from build123d import *

# Parameters (mm, degrees)
SKETCH1_W           = 70
SKETCH1_H           = 41
BOSS_EXTRUDE1_DEPTH = 12
SKETCH2_W           = 50
SKETCH2_H           = 1
CUT_EXTRUDE1_DEPTH  = 88
SKETCH3_R           = 2.5
SKETCH3_R_2         = 2.75
CUT_EXTRUDE2_DEPTH  = 88
SKETCH4_R           = 5
CUT_EXTRUDE3_DEPTH  = 5.7
SKETCH5_R           = 2.5
CUT_EXTRUDE4_DEPTH  = 12
SKETCH6_R           = 6
SKETCH6_R_2         = 5.5
CUT_EXTRUDE5_DEPTH  = 39
SKETCH8_R           = 2.5
BOSS_EXTRUDE2_DEPTH = 41
SKETCH9_R           = 2.5
CUT_EXTRUDE6_DEPTH  = 12
SKETCH10_R          = 6
CUT_EXTRUDE7_DEPTH  = 30


with BuildPart() as part:
    # Sketch1 → Boss-Extrude1 (new body)
    with BuildSketch(Plane(origin=(0, 0, 0), x_dir=(1, 0, 0), z_dir=(0, 1, 0))):
        Rectangle(SKETCH1_W, SKETCH1_H)
    extrude(amount=BOSS_EXTRUDE1_DEPTH)

    # Sketch2 → Cut-Extrude1 (cut)
    with BuildSketch(Plane.XY.offset(20.5)):
        with Locations((0, 11.5)):
            Rectangle(SKETCH2_W, SKETCH2_H)
    extrude(amount=-CUT_EXTRUDE1_DEPTH, mode=Mode.SUBTRACT)

    # Sketch3 → Cut-Extrude2 (cut)
    with BuildSketch(Plane.XZ):
        with Locations((29, -7.5)):
            Circle(SKETCH3_R)
        with Locations((-29, 7.5)):
            Circle(SKETCH3_R)
        with Locations((29, 7.5)):
            Circle(SKETCH3_R_2)
        with Locations((-29, -7.5)):
            Circle(SKETCH3_R_2)
    extrude(amount=-CUT_EXTRUDE2_DEPTH, mode=Mode.SUBTRACT)

    # Sketch4 → Cut-Extrude3 (cut)
    with BuildSketch(Plane.XZ):
        with Locations((-29, -7.5)):
            Circle(SKETCH4_R)
        with Locations((29, 7.5)):
            Circle(SKETCH4_R)
    extrude(amount=-CUT_EXTRUDE3_DEPTH, mode=Mode.SUBTRACT)

    # Sketch5 → Cut-Extrude4 (cut)
    with BuildSketch(Plane(origin=(0, 0, -20.5), x_dir=(-1, 0, 0), z_dir=(0, 0, -1))):
        with Locations((-6.5, 6)):
            Circle(SKETCH5_R)
    extrude(amount=-CUT_EXTRUDE4_DEPTH, mode=Mode.SUBTRACT)

    # Sketch6 → Cut-Extrude5 (cut)
    with BuildSketch(Plane.XZ):
        Circle(SKETCH6_R)
        with Locations((-17.5, 0)):
            Circle(SKETCH6_R_2)
        with Locations((17.5, 0)):
            Circle(SKETCH6_R_2)
    extrude(amount=-CUT_EXTRUDE5_DEPTH, mode=Mode.SUBTRACT)

    # Sketch8 → Boss-Extrude2 (add)
    with BuildSketch(Plane(origin=(0, 0, -20.5), x_dir=(-1, 0, 0), z_dir=(0, 0, -1))):
        with Locations((-6.5, 6)):
            Circle(SKETCH8_R)
    extrude(amount=-BOSS_EXTRUDE2_DEPTH)

    # Sketch9 → Cut-Extrude6 (cut)
    with BuildSketch(Plane(origin=(0, 0, -20.5), x_dir=(-1, 0, 0), z_dir=(0, 0, -1))):
        with Locations((-6.5, 5.5)):
            Circle(SKETCH9_R)
    extrude(amount=-CUT_EXTRUDE6_DEPTH, mode=Mode.SUBTRACT)

    # Sketch10 → Cut-Extrude7 (cut)
    with BuildSketch(Plane(origin=(0, 11, 0), x_dir=(1, 0, 0), z_dir=(0, 1, 0))):
        Circle(SKETCH10_R)
    extrude(amount=-CUT_EXTRUDE7_DEPTH, mode=Mode.SUBTRACT)


solid = part.part
The listing builds one solid part. Answer for the finished solid, in the listing's coordinates (mm). A direction names the side the tool comes from. Give positions to 0.01 mm unless a question says otherwise; leave off trailing zeros. Loops run counter-clockwise (first coordinate to the right, second up) from the corner with the lowest first, then second, coordinate; pieces in that order, holes last. Notation, with made-up numbers: (36, 3.5) - (66, 3.5) arc R22 ccw to (66, 29.5) - close; hole circle Ø4 at (24.5, 24.5). An arc over 180 degrees is marked (long way). Answer as a JSON object with one key per item and string values.
1. A cutting plane is placed at B-B (y = 9.25). Write down the section's boundary in (x, z), then the cut area to 3 significant figures.
Determined:
{"outline": "(-35, -20.5) - (35, -20.5) - (35, 20.5) - (-35, 20.5) - close; hole circle Ø5.5 at (-29, -7.5); hole circle Ø5 at (-29, 7.5); hole circle Ø11 at (-17.5, 0); hole circle Ø12 at (0, 0); hole circle Ø11 at (17.5, 0); hole circle Ø5.5 at (29, 7.5); hole circle Ø5 at (29, -7.5)", "area": "2,480 mm²"}
2. For a pull along Y with two mould halves and no side action, classify faces 3 (the cylindrical face through (4.115, 6.251, -14.584)), 4 (the flat face through (7, 6, -8.5)), 5 (the flat face through (-6, 11, 5)), 6 (the cylindrical face through (26.253, 8.806, 7.621)) as pulls with the +Y half, pulls with the -Y half, needs draft (parallel to the pull), parting line crosses it, or undercut.
Determined:
{"face 3": "undercut", "face 4": "undercut", "face 5": "pulls with the +Y half", "face 6": "needs draft"}
3. A cutting plane is placed at A-A (x = -29). Write down the section's boundary in (y, z), then the cut area to 3 significant figures.
Determined:
{"outline": "(0, -20.5) - (12, -20.5) - (12, -10.25) - (5.7, -10.25) - (5.7, -12.5) - (0, -12.5) - close; (0, -2.5) - (5.7, -2.5) - (5.7, -4.75) - (12, -4.75) - (12, 5) - (0, 5) - close; (0, 10) - (12, 10) - (12, 20.5) - (0, 20.5) - close", "area": "340 mm²"}
4. A cutting plane is placed at C-C (z = 0). Write down the section's boundary in (x, y).
Determined:
{"outline": "(-35, 0) - (-23, 0) - (-23, 11) - (-25, 11) - (-25, 12) - (-35, 12) - close; (-12, 0) - (-6, 0) - (-6, 11) - (-12, 11) - close; (6, 0) - (12, 0) - (12, 11) - (6, 11) - close; (23, 0) - (35, 0) - (35, 12) - (25, 12) - (25, 11) - (23, 11) - close"}
5. For faces 1 (the flat face through (30, 12, 0)), 2 (the flat face through (-27, 5.7, -10)), determine the directions among +Z, -Z, +X, -X, +Y, -Y from which every point of the face is accessible in a straight line to the end or side of a thin tool.
Determined:
{"face 1": "+Z, -Z, +X, -X, +Y", "face 2": "-Y"}
6. Flat-ended cylindrical pins translate along their axes: pin 1 Ø6 at (x, z) = (-12, -13.5) entering from +Y; pin 2 Ø8 at (x, z) = (-29.5, -7.5) entering from -Y. Find the tip coordinate at first contact, or state that the pin passes through.
Determined:
{"pin 1": "y = 11", "pin 2": "y = 5.7"}
7. A cutting plane is placed at D-D (x = 17.5). Write down the section's boundary in (y, z).
Determined:
{"outline": "(0, -20.5) - (11, -20.5) - (11, -5.5) - (0, -5.5) - close; (0, 5.5) - (11, 5.5) - (11, 20.5) - (0, 20.5) - close"}
8. Find the intervals of material crossed by L1, parallel to Z at x = -29, y = 8.75; L2, parallel to X at y = 9.75, z = -8.5; L3, parallel to Y at x = -22, z = 11, in increasing order. Write a range as [from, to].
Determined:
{"L1": "[-20.5, -10.25], [-4.75, 5], [10, 20.5]", "L2": "[-35, -31.56], [-26.44, 26.71], [31.29, 35]", "L3": "[0, 11]"}
